```python
from build123d import *

# Parameters (mm, degrees)
F0_R     = 4.25
F0_R_2   = 44
F1_DEPTH = 2.5
F2_R     = 5


with BuildPart() as f1:
    # F0 (on Top) → F1 (new body)
    with BuildSketch(Plane.XY):
        with BuildLine():
            Line((85, 10.5), (65.1594198869, 10.5))
            ThreePointArc((65.1594198869, 10.5), (-66, 0), (65.1594198869, -10.5))
            Line((65.1594198869, -10.5), (85, -10.5))
            Line((85, -10.5), (85, 10.5))
        make_face()
        with Locations((38.8817437881, -38.9)):
            Circle(F0_R, mode=Mode.SUBTRACT)
        with Locations((-55, 0)):
            Circle(F0_R, mode=Mode.SUBTRACT)
        Circle(F0_R_2, mode=Mode.SUBTRACT)
        with Locations((38.8817437881, 38.9)):
            Circle(F0_R, mode=Mode.SUBTRACT)
    extrude(amount=F1_DEPTH)

    # F2
    f2_edges = [f1.edges().sort_by_distance(p)[0] for p in [
        (65.15942, 10.5, 1.25),
        (65.15942, -10.5, 1.25),
    ]]
    fillet(f2_edges, radius=F2_R)


solid = f1.part
```
Design review of the part built by this model. Coordinates are the model's own, in mm. Round coordinates to 2 decimals unless told otherwise and drop trailing zeros. Write each loop counter-clockwise with the first axis right and the second up, starting at its lowest first coordinate (ties: lowest second). Pieces come first, ordered by that corner, then holes. Notation, with made-up numbers: (84, 27) -> (125, 27) arc R18 cw to (125, 59) -> close; hole circle Ø6 at (55.5, 57.25). An arc over 180 degrees is marked (long way). Answer in a Markdown table with one row per item.
Q1. Take a section at C-C, the plane y = 22. State the section outline as (x, z) points.
The answers:
| item | result |
|---|---|
| outline | (-62.23, 0) -> (-38.11, 0) -> (-38.11, 2.5) -> (-62.23, 2.5) -> close; (38.11, 0) -> (62.23, 0) -> (62.23, 2.5) -> (38.11, 2.5) -> close |
Q2. Take a section at D-D, the plane x = -38.5. State the section outline as (y, z) points, then the cut area to 3 significant figures.
The answers:
| item | result |
|---|---|
| outline | (-53.61, 0) -> (-21.3, 0) -> (-21.3, 2.5) -> (-53.61, 2.5) -> close; (21.3, 0) -> (53.61, 0) -> (53.61, 2.5) -> (21.3, 2.5) -> close |
| area | 162 mm² |
Q3. Draft analysis for pull direction X (two halves, no side actions). For faces 1 (the face through (66.199, 11.568, 1.268)), 2 (the face through (42, 16, 0)), 3 (the face through (42.808, 37.272, 1.232)), state which applies: +X half, -X half, draft (parallel to the pull), parting line (faces both ways), or undercut.
The answers:
| item | result |
|---|---|
| face 1 | +X half |
| face 2 | draft |
| face 3 | undercut |
Q4. Clearance check with flat-ended pins moving along their axes: pin 1 Ø1.5 at (y, z) = (47, 1) entering from -X; pin 2 Ø11 at (x, y) = (38.88, -38.9) entering from +Z; pin 3 Ø1 at (y, z) = (16, 2) entering from +X; pin 4 Ø7.5 at (x, y) = (38.88, 38.9) entering from -Z. State where each tip first meets the part, or that it passes through.
The answers:
| item | result |
|---|---|
| pin 1 | x = -47.08 |
| pin 2 | z = 2.5 |
| pin 3 | x = 64.15 |
| pin 4 | through |
Q5. Take a section at A-A, the plane y = 0. State the section outline as (x, z) points.
The answers:
| item | result |
|---|---|
| outline | (-66, 0) -> (-59.25, 0) -> (-59.25, 2.5) -> (-66, 2.5) -> close; (-50.75, 0) -> (-44, 0) -> (-44, 2.5) -> (-50.75, 2.5) -> close; (44, 0) -> (85, 0) -> (85, 2.5) -> (44, 2.5) -> close |
Q6. Take a section at B-B, the plane z = 2. State the section outline as (x, y) points.
The answers:
| item | result |
|---|---|
| outline | (64.41, -14.41) arc R5 cw to (69.29, -10.5) -> (85, -10.5) -> (85, 10.5) -> (69.29, 10.5) arc R5 cw to (64.41, 14.41) arc R66 ccw (long way) to start; hole circle Ø8.5 at (-55, 0); hole circle Ø88 at (0, 0); hole circle Ø8.5 at (38.88, -38.9); hole circle Ø8.5 at (38.88, 38.9) |
Q7. To check wall thickness, follow L1, parallel to X at y = -38, z = 1.25; L2, parallel to X at y = -3.5, z = 2.2; L3, parallel to X at y = 12, z = 0.7. State the ranges of each line that lie inside material, in increasing order. Write a range as [from, to].
The answers:
| item | result |
|---|---|
| L1 | [-53.96, -22.18], [22.18, 34.73], [43.04, 53.96] |
| L2 | [-65.91, -57.41], [-52.59, -43.86], [43.86, 85] |
| L3 | [-64.9, -42.33], [42.33, 65.72] |
